```python
from build123d import *

# Parameters (mm, degrees)
SKETCH1_R            = 4.25
BASE_FLANGE1_DEPTH   = 2
FILLET1_R            = 20
M5_CLEARANCE_HOLE1_D = 5.5
FILLET2_R            = 4


# Sheet-metal steps are written as plain solids
with BuildPart() as part:
    # Sketch1 → Base-Flange1 (new body)
    with BuildSketch(Plane(origin=(0, 0, 0), x_dir=(1, 0, 0), z_dir=(0, 1, 0))):
        with BuildLine():
            Line((-10, 0), (10, 0))
            Line((10, 0), (10, 26))
            Line((10, 26), (14.871793605, 41.530715601))
            ThreePointArc((14.871793605, 41.530715601), (9.910471049, 51.719563347), (-0.542628251, 47.342343349))
            Line((-0.542628251, 47.342343349), (-10, 26))
            Line((-10, 26), (-10, 0))
        make_face()
        with Locations(Location((7, 44, 0), (0, 0, 270))):
            Circle(SKETCH1_R, mode=Mode.SUBTRACT)
    extrude(amount=-BASE_FLANGE1_DEPTH)

    # Fillet1
    fillet1_edges = [part.edges().sort_by_distance(p)[0] for p in [
        (-10, -1, -26),
        (10, -1, -26),
    ]]
    fillet(fillet1_edges, radius=FILLET1_R)

    # M5 Clearance Hole1 (through all)
    with Locations(Plane(origin=(0, 0, 0), x_dir=(1, 0, 0), z_dir=(0, 1, 0))):
        with Locations((0, 16), (0, 5)):
            Hole(M5_CLEARANCE_HOLE1_D / 2)

    # Fillet2
    fillet2_edges = [part.edges().sort_by_distance(p)[0] for p in [
        (10, -1, 0),
        (-10, -1, 0),
    ]]
    fillet(fillet2_edges, radius=FILLET2_R)


solid = part.part
```
CAD build for the part. Positions are in the model's coordinates, mm. A direction names the side the tool comes from. Round coordinates to 2 decimals unless told otherwise and drop trailing zeros. Write each loop counter-clockwise with the first axis right and the second up, starting at its lowest first coordinate (ties: lowest second). Pieces come first, ordered by that corner, then holes.
Item 1: Band-saw the part on D-D on x = 0. Write the cut outline in (y, z), then the cut area to 3 significant figures.
Filled in:
outline: (-2, -48.37) - (0, -48.37) - (0, -18.75) - (-2, -18.75) - close; (-2, -13.25) - (0, -13.25) - (0, -7.75) - (-2, -7.75) - close; (-2, -2.25) - (0, -2.25) - (0, 0) - (-2, 0) - close
area: 74.7 mm2
Item 2: Mould opens along X. For faces 3 (the flat face through (2, -2, -26)), 4 (the cylindrical face through (0.596, -1.014, -2.315)), 5 (the cylindrical face through (0.358, -1.014, -18.727)), 6 (the cylindrical face through (10.073, -0.986, -51.656)) say: released by +X, released by -X, zero draft, split by the parting line, or undercut.
Filled in:
face 3: zero draft
face 4: undercut
face 5: undercut
face 6: split by the parting line
Item 3: Drop a flat-ended pin along its axis: pin 1 Ø5 at (x, z) = (0, -5) entering from -Y. Give the stop position or say it passes through.
Filled in:
pin 1: passes through
Item 4: Drill centre lines: L1, parallel to Z at x = -1, y = -0.05; L2, parallel to Z at x = 0, y = -0.55; L3, parallel to X at y = -0.35, z = -8. Where is each one in solid material? Low to high.
Filled in:
L1: z = -46.31 to -18.56, -13.44 to -7.56, -2.44 to 0
L2: z = -48.37 to -18.75, -13.25 to -7.75, -2.25 to 0
L3: x = -10 to 10
Item 5: Band-saw the part on B-B on x = 7.75. Write the cut outline in (y, z).
Filled in:
outline: (-2, -52.22) - (0, -52.22) - (0, -48.18) - (-2, -48.18) - close; (-2, -39.82) - (0, -39.82) - (0, -0.4) - (-2, -0.4) - close
Item 6: Band-saw the part on C-C on y = -1.15. Write the cut outline in (x, z).
Filled in:
outline: (-10, -21.77) arc R20 ccw to (-8.29, -29.87) - (-0.54, -47.34) arc R8.25 ccw to (14.87, -41.53) - (10.92, -28.92) arc R20 cw to (10, -22.94) - (10, -4) arc R4 ccw to (6, 0) - (-6, 0) arc R4 ccw to (-10, -4) - close; hole circle Ø5.5 at (0, -16); hole circle Ø5.5 at (0, -5); hole circle Ø8.5 at (7, -44)
Item 7: Tool access for faces 1 (the flat face through (10, -1, -13)), 2 (the cylindrical face through (-9.58, -1.01, -25.85)): list every direction of +Z, -Z, +X, -X, +Y, -Y with a clear straight run to the whole face (end or side of a thin tool).
Filled in:
face 1: +Z, +X, +Y, -Y
face 2: -Z, -X, +Y, -Y
Item 8: Band-saw the part on A-A on z = -16. Write the cut outline in (x, y), then the cut area to 3 significant figures.
Filled in:
outline: (-10, -2) - (-2.75, -2) - (-2.75, 0) - (-10, 0) - close; (2.75, -2) - (10, -2) - (10, 0) - (2.75, 0) - close
area: 29.0 mm2
